Design review of the part shown in the three views and the two pictorial views. Dimensions are in mm from the part's minimum x, y and z. A direction names the side the tool comes from. Round coordinates to 2 decimals unless told otherwise and drop trailing zeros. Loops run counter-clockwise (first coordinate to the right, second up) from the corner with the lowest first, then second, coordinate; pieces in that order, holes last. Notation, with made-up numbers: (-16, 27) -> (37, 27) arc R15 cw to (37, 54) -> close; hole circle Ø3 at (52, 64.25). An arc over 180 degrees is marked (long way). Use CSV: the item, a comma, the result in double quotes. Start each with the question number.
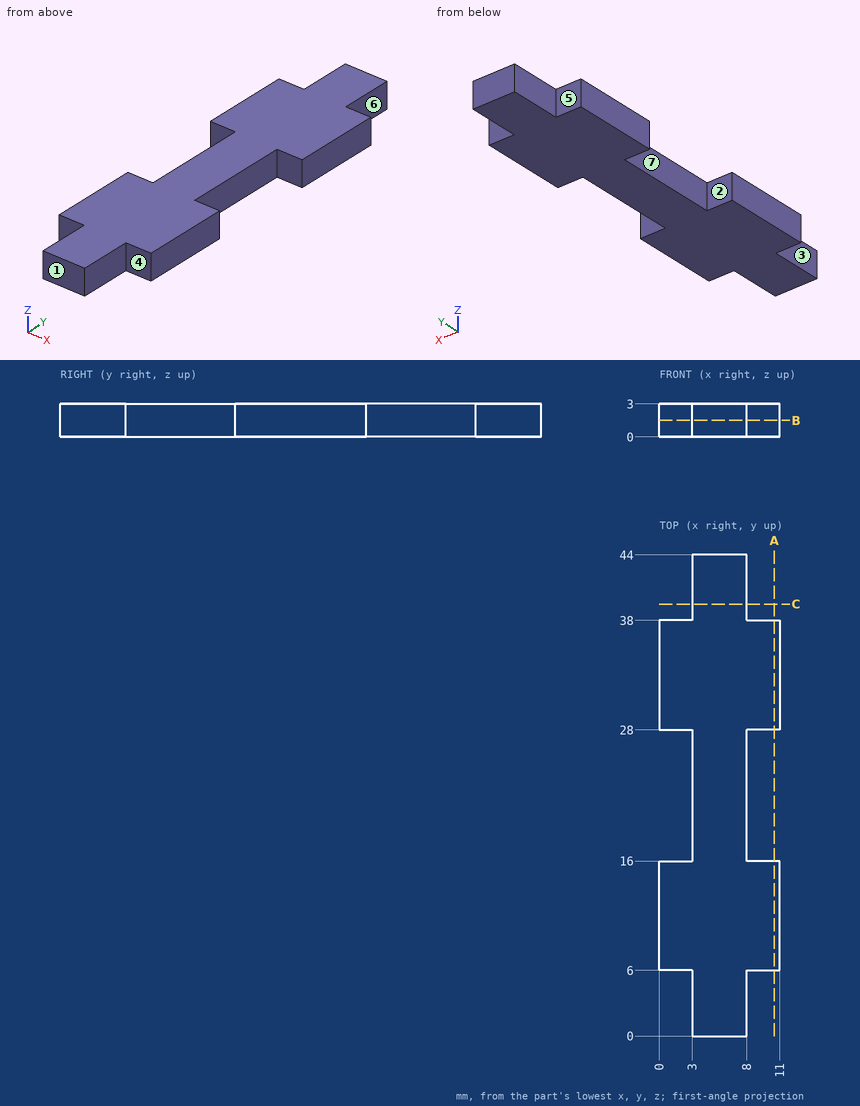
1. Take a section at B-B, the plane z = 1.5. Give the boundary of the cut face in (x, y), then the cut area to 3 significant figures.
2. Take a section at A-A, the plane x = 10.5. Give the boundary of the cut face in (y, z).
3. Clearance check with flat-ended pins moving along their axes: P1, Ø0.9, axis at x = 1.5, z = 1, coming from the -Y side; P2, Ø0.9, axis at y = 3, z = 2, coming from the -X side; P3, Ø0.9, axis at y = 21.5, z = 2, coming from the +X side. State where each tip first meets the part, or that it passes through.
4. The part is to be moulded in two halves that separate along Y. For the marked faces 1, 2 and 3, say which applies: pulls with the +Y half, pulls with the -Y half, needs draft (parallel to the pull), parting line crosses it, or undercut.
5. For line 1 along Y through (x, z) = (9, 2.45); line 2 along X through (y, z) = (5, 2.5), list the stretches that pass through material, from the lowest coordinate up. Write a range as from..to.
6. For the marked faces 4, 5, 6 and 7, list the 3-axis set-ups (+Z, -Z, +X, -X, +Y, -Y) from which the entire face can be reached by the end or side of a thin tool; tool diameter is ignored.
7. Take a section at C-C, the plane y = 39.5. Give the boundary of the cut face in (x, z), then the cut area to 3 significant figures.
Results:
1,outline,"(0, 6) -> (3, 6) -> (3, 0) -> (8, 0) -> (8, 6) -> (11, 6) -> (11, 16) -> (8, 16) -> (8, 28) -> (11, 28) -> (11, 38) -> (8, 38) -> (8, 44) -> (3, 44) -> (3, 38) -> (0, 38) -> (0, 28) -> (3, 28) -> (3, 16) -> (0, 16) -> close"
1,area,"340 mm²"
2,outline,"(6, 0) -> (16, 0) -> (16, 3) -> (6, 3) -> close; (28, 0) -> (38, 0) -> (38, 3) -> (28, 3) -> close"
3,P1,"y = 6"
3,P2,"x = 3"
3,P3,"x = 8"
4,face 1,"pulls with the -Y half"
4,face 2,"undercut"
4,face 3,"needs draft"
5,line 1,"6..16, 28..38"
5,line 2,"3..8"
6,face 4,"+Z, -Z, +X, -Y"
6,face 5,"+Z, -Z, -X, +Y"
6,face 6,"+Z, -Z, +X, +Y"
6,face 7,"+Z, -Z, -X"
7,outline,"(3, 0) -> (8, 0) -> (8, 3) -> (3, 3) -> close"
7,area,"15.0 mm²"
